from build123d import *

# Parameters (mm, degrees)
EXTRUDE1_START     = 7
EXTRUDE1_DEPTH     = 20
SKETCH2_R          = 7.5
CUT_EXTRUDE1_DEPTH = 2
SHELL1_START       = 7
SHELL1_DEPTH       = 18
EXTRUDE2_DEPTH     = 12
SKETCH9_R          = 3
EXTRUDE4_DEPTH     = 1.38
SKETCH10_R         = 2.5
CUT_EXTRUDE3_DEPTH = 49.252462113
FILLET1_R          = 0.2
SKETCH11_W         = 36
SKETCH11_H         = 46
SKETCH11_W_2       = 32
SKETCH11_H_2       = 42
EXTRUDE5_DEPTH     = 6
SKETCH12_W         = 32
SKETCH12_H         = 8.201060756
CUT_EXTRUDE4_DEPTH = 2
SKETCH13_W         = 36
SKETCH13_H         = 32
EXTRUDE6_DEPTH     = 2


# Read off the part's stored shape, not the designer's step: Shell1
with BuildPart() as part:
    # Sketch1 → Extrude1 (new body)
    with BuildSketch(Plane.XY.offset(EXTRUDE1_START)):
        with BuildLine():
            Line((-7.266188822, -9.55), (7.266188822, -9.55))
            ThreePointArc((7.266188822, -9.55), (12, 0), (7.266188822, 9.55))
            Line((7.266188822, 9.55), (-7.266188822, 9.55))
            ThreePointArc((-7.266188822, 9.55), (-12, 0), (-7.266188822, -9.55))
        make_face()
    extrude(amount=EXTRUDE1_DEPTH)

    # Sketch2 → Cut-Extrude1 (cut)
    with BuildSketch(Plane.XY.offset(27)):
        Circle(SKETCH2_R)
    extrude(amount=-CUT_EXTRUDE1_DEPTH, mode=Mode.SUBTRACT)

    # Shell1 outline → Shell1 (cut)
    with BuildSketch(Plane.XY.offset(SHELL1_START)):
        with BuildLine():
            Line((6.557247898, 7.55), (-6.557247898, 7.55))
            ThreePointArc((-6.557247898, 7.55), (-10, 0), (-6.557247898, -7.55))
            Line((-6.557247898, -7.55), (6.557247898, -7.55))
            ThreePointArc((6.557247898, -7.55), (10, 0), (6.557247898, 7.55))
        make_face()
    extrude(amount=SHELL1_DEPTH, mode=Mode.SUBTRACT)

    # Sketch5 → Extrude2 (add)
    with BuildSketch(Plane.XY.offset(27)):
        with BuildLine():
            Line((-7.266188822, -9.55), (7.266188822, -9.55))
            ThreePointArc((7.266188822, -9.55), (10.751610713, -5.329434029), (12, 0))
            Line((12, 0), (12, 9.55))
            Line((12, 9.55), (10, 9.55))
            Line((10, 9.55), (10, 0))
            ThreePointArc((10, 0), (9.098694384, -4.148946916), (6.557247898, -7.55))
            Line((6.557247898, -7.55), (-6.557247898, -7.55))
            ThreePointArc((-6.557247898, -7.55), (-9.098694384, -4.148946916), (-10, 0))
            Line((-10, 0), (-10, 9.55))
            Line((-10, 9.55), (-12, 9.55))
            Line((-12, 9.55), (-12, 0))
            ThreePointArc((-12, 0), (-10.751610713, -5.329434029), (-7.266188822, -9.55))
        make_face()
    extrude(amount=EXTRUDE2_DEPTH)

    # Sketch9 → Extrude4 (add)
    with BuildSketch(Plane(origin=(12, 0, 0), x_dir=(0, 0, -1), z_dir=(1, 0, 0))):
        with Locations(Location((-33, 5, 0), (0, 0, 180))):
            Circle(SKETCH9_R)
    extrude4 = extrude(amount=EXTRUDE4_DEPTH)

    # Mirror2: Extrude4 across plane
    add(extrude4.mirror(Plane(origin=(0, 0, 0), x_dir=(0, 0, 1), z_dir=(1, 0, 0))))

    # Sketch10 → Cut-Extrude3 (cut, through all)
    with BuildSketch(Plane(origin=(13.38, 0, 0), x_dir=(0, 0, -1), z_dir=(1, 0, 0))):
        with Locations((-33, 5)):
            Circle(SKETCH10_R)
    extrude(amount=-CUT_EXTRUDE3_DEPTH, mode=Mode.SUBTRACT)

    # Fillet1
    fillet1_edges = [part.edges().sort_by_distance(p)[0] for p in [
        (-13.38, 5, 35.5),
        (13.38, 5, 35.5),
    ]]
    fillet(fillet1_edges, radius=FILLET1_R)



with BuildPart() as body_2:
    # Sketch11 → Extrude5 (new body)
    with BuildSketch(Plane.XZ.offset(9.55)):
        with Locations((0, 23)):
            Rectangle(SKETCH11_W, SKETCH11_H)
        with Locations((0, 23)):
            Rectangle(SKETCH11_W_2, SKETCH11_H_2, mode=Mode.SUBTRACT)
    extrude(amount=EXTRUDE5_DEPTH)

    # Sketch12 → Cut-Extrude4 (cut)
    with BuildSketch(Plane(origin=(0, 0, 0), x_dir=(-1, 0, 0), z_dir=(0, 0, -1))):
        with Locations((0, -12.325842128)):
            Rectangle(SKETCH12_W, SKETCH12_H)
    extrude(amount=-CUT_EXTRUDE4_DEPTH, mode=Mode.SUBTRACT)


with BuildPart() as part_1:
    add(part.part)

    add(body_2.part)  # Extrude6 merges body 2
    # Sketch13 → Extrude6 (add)
    with BuildSketch(Plane.XZ.offset(9.55)):
        with Locations((0, 23)):
            Rectangle(SKETCH13_W, SKETCH13_H)
    extrude(amount=-EXTRUDE6_DEPTH)


solid = part_1.part
Here's how the part is built. I have some questions about the finished solid (model axes, mm). A direction names the side the tool comes from. Give positions to 0.01 mm unless a question says otherwise; leave off trailing zeros. Write each loop counter-clockwise with the first axis right and the second up, starting at its lowest first coordinate (ties: lowest second). Pieces come first, ordered by that corner, then holes. Notation, with made-up numbers: (8, 0.5) -> (37, 0.5) arc R24 ccw to (37, 14.5) -> close; hole circle Ø3 at (78, 45). An arc over 180 degrees is marked (long way). Use one line per item in the form item = value. Start each with the question number.
1. Thinking about a two-plate mould opening in X: for faces 5 (the face through (-18, -12, 23)), 6 (the face through (9.123, -4.094, 32.916)), 7 (the face through (-17, -9.55, 4)), which applies, +X half, -X half, draft (parallel to the pull), parting line (faces both ways), or undercut?
2. Imagine slicing it at D-D on x = 11. List the corners of the cut face in (y, z) for me, plus the area to 3 significant figures.
3. Imagine slicing it at A-A on z = 12. List the corners of the cut face in (x, y) for me, plus the area to 3 significant figures.
4. Imagine slicing it at C-C on y = -3.5. List the corners of the cut face in (x, z) for me, plus the area to 3 significant figures.
5. On a 3-axis mill with a long thin cutter (end or side, diameter ignored), from which of +Z, -Z, +X, -X, +Y, -Y can I reach the whole of each face in a straight line? I mean faces 1 (the face through (16, -13, 22)), 2 (the face through (4, 7, 27)), 3 (the face through (-14, -7.55, 23)), 4 (the face through (0, 7.55, 16)). Say none if no direction works.
6. Imagine slicing it at B-B on x = 0. List the corners of the cut face in (y, z) for me, plus the area to 3 significant figures.
7. Will these pins go through, and if not, where does the flat tip stop? pin 1 Ø10 at (x, z) = (9, 37.5) entering from -Y; pin 2 Ø3 at (y, z) = (3, 36) entering from -X; pin 3 Ø5 at (y, z) = (5.5, 36) entering from +X.
8. If I drill on L1, parallel to Y at x = -12.45, z = 33; L2, parallel to X at y = -10, z = 13; L3, parallel to X at y = 1, z = 29, over which ranges is the centre line in solid material (lowest first)?
Entries:
q1.face_5 = -X half
q1.face_6 = undercut
q1.face_7 = draft
q2.outline = (-15.55, 44) -> (-9.55, 44) -> (-9.55, 46) -> (-15.55, 46) -> close; (-9.55, 7) -> (-7.55, 7) -> (-7.55, 39) -> (-9.55, 39) -> close; (-4.8, 7) -> (4.8, 7) -> (4.8, 27) -> (9.55, 27) -> (9.55, 39) -> (-4.8, 39) -> close; hole circle Ø5 at (5, 33)
q2.area = 420 mm²
q3.outline = (-18, -15.55) -> (-16, -15.55) -> (-16, -9.55) -> (16, -9.55) -> (16, -15.55) -> (18, -15.55) -> (18, -7.55) -> (9.33, -7.55) arc R12 ccw to (7.27, 9.55) -> (-7.27, 9.55) arc R12 ccw to (-9.33, -7.55) -> (-18, -7.55) -> close; hole (-6.56, -7.55) -> (6.56, -7.55) arc R10 ccw to (6.56, 7.55) -> (-6.56, 7.55) arc R10 ccw to start
q3.area = 196 mm²
q4.outline = (-11.48, 7) -> (-9.37, 7) -> (-9.37, 25) -> (-6.63, 25) -> (-6.63, 27) -> (-9.37, 27) -> (-9.37, 39) -> (-11.48, 39) -> close; (6.63, 25) -> (9.37, 25) -> (9.37, 7) -> (11.48, 7) -> (11.48, 39) -> (9.37, 39) -> (9.37, 27) -> (6.63, 27) -> close
q4.area = 146 mm²
q5.face_1 = -Z, -Y
q5.face_2 = +Z, +Y
q5.face_3 = +Z, -Z, -X
q5.face_4 = -Z
q6.outline = (-15.55, 44) -> (-9.55, 44) -> (-9.55, 46) -> (-15.55, 46) -> close; (-9.55, 7) -> (-7.55, 7) -> (-7.55, 25) -> (-7.5, 25) -> (-7.5, 27) -> (-7.55, 27) -> (-7.55, 39) -> (-9.55, 39) -> close; (7.5, 25) -> (7.55, 25) -> (7.55, 7) -> (9.55, 7) -> (9.55, 27) -> (7.5, 27) -> close
q6.area = 116 mm²
q7.pin_1 = -9.55
q7.pin_2 = -13.38
q7.pin_3 = 13.38
q8.L1 = -9.55 to -7.55, 2 to 2.5, 7.5 to 8
q8.L2 = -18 to -16, 16 to 18
q8.L3 = -12 to -10, 10 to 12
